Check sheet for the modelled part. Datum: model origin and axes. Units: mm. Face numbers are marked on the shaded views. A direction names the side the tool comes from. Give positions to 0.01 mm unless a question says otherwise; leave off trailing zeros. Order: outer loops, then holes, each group sorted by start corner. A loop starts at its lowest first (then second) coordinate and runs counter-clockwise, first axis right, second up.
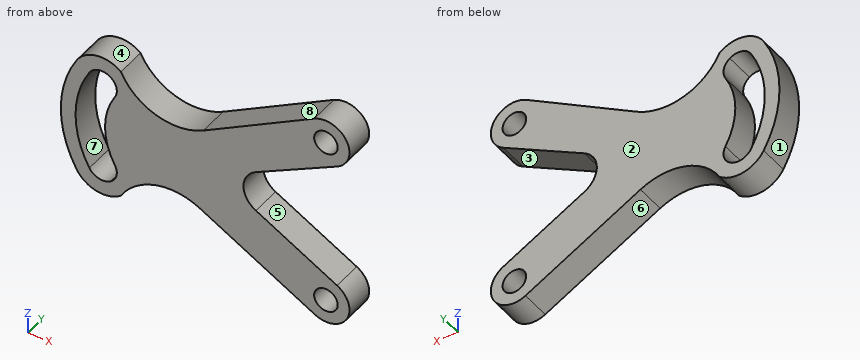
from build123d import *

# Parameters (mm, degrees)
F0_R     = 10
F1_DEPTH = 25


with BuildPart() as f1:
    # F0 (on Front) → F1 (new body)
    with BuildSketch(Plane.XZ):
        with BuildLine():
            Line((65.554609, 17.629084), (134.445391, 54.5397))
            ThreePointArc((134.445391, 54.5397), (142.476996, 81.892703), (115, 89.489292))
            Line((115, 89.489292), (21.000572, 35.218697))
            ThreePointArc((21.000572, 35.218697), (-18.704666, 30.731307), (-49.0183, 56.764481))
            ThreePointArc((-49.0183, 56.764481), (-69.380297, 62.104661), (-86.60254, 50))
            ThreePointArc((-86.60254, 50), (-100, 0), (-86.60254, -50))
            ThreePointArc((-86.60254, -50), (-69.380297, -62.104661), (-49.0183, -56.764481))
            ThreePointArc((-49.0183, -56.764481), (-19.419281, -33.5396), (17.992089, -37.525377))
            Line((17.992089, -37.525377), (115.554609, -89.797867))
            ThreePointArc((115.554609, -89.797867), (142.629084, -81.614174), (134.445391, -54.5397))
            Line((134.445391, -54.5397), (65.554609, -17.629084))
            ThreePointArc((65.554609, -17.629084), (55, 0), (65.554609, 17.629084))
        make_face()
        with BuildLine():
            ThreePointArc((-75.777223, 43.75), (-67.680804, 49.698488), (-57.821535, 47.766831))
            ThreePointArc((-57.821535, 47.766831), (-52.753417, 40.228899), (-54.126588, 31.25))
            ThreePointArc((-54.126588, 31.25), (-62.5, 0), (-54.126588, -31.25))
            ThreePointArc((-54.126588, -31.25), (-52.753417, -40.228899), (-57.821535, -47.766831))
            ThreePointArc((-57.821535, -47.766831), (-67.680804, -49.698488), (-75.777223, -43.75))
            ThreePointArc((-75.777223, -43.75), (-87.5, 0), (-75.777223, 43.75))
        make_face(mode=Mode.SUBTRACT)
        with Locations((125, -72.168784)):
            Circle(F0_R, mode=Mode.SUBTRACT)
        with Locations((125, 72.168784)):
            Circle(F0_R, mode=Mode.SUBTRACT)
    extrude(amount=F1_DEPTH)


solid = f1.part
1) Depth check by flat-ended pin: pin 1 Ø12 at (y, z) = (-21, 52) entering from -X; pin 2 Ø1.5 at (y, z) = (-9.5, 31) entering from -X; pin 3 Ø3 at (x, y) = (-52.5, -10.5) entering from +Z. Enter the tip coordinate at first touch or a pass-through.
Recorded:
pin 1: stops at x = -88.79
pin 2: stops at x = -95.31
pin 3: stops at z = 59.97
2) Section check D-D, the plane x = 27. Record the cut outline in (y, z), then the cut area to 3 significant figures.
Recorded:
outline: (-25, -42.35) - (0, -42.35) - (0, 38.68) - (-25, 38.68) - close
area: 2,030 mm2
3) Section check C-C, the plane x = 70. Record the cut outline in (y, z), then the cut area to 3 significant figures.
Recorded:
outline: (-25, -65.39) - (0, -65.39) - (0, -20.01) - (-25, -20.01) - close; (-25, 20.01) - (0, 20.01) - (0, 63.51) - (-25, 63.51) - close
area: 2,220 mm2
4) Section check B-B, the plane y = -9.75. Record the cut outline in (x, z), then the cut area to 3 significant figures.
Recorded:
outline: (-86.6, -50) arc R25 ccw to (-49.02, -56.76) arc R50 cw to (17.99, -37.53) - (115.55, -89.8) arc R20 ccw to (134.45, -54.54) - (65.55, -17.63) arc R20 cw to (65.55, 17.63) - (134.45, 54.54) arc R20 ccw (long way) to (115, 89.49) - (21, 35.22) arc R50 cw to (-49.02, 56.76) arc R25 ccw to (-86.6, 50) arc R100 ccw to start; hole (-75.78, -43.75) arc R12.5 ccw to (-57.82, -47.77) arc R12.5 ccw to (-54.13, -31.25) arc R62.5 cw to (-54.13, 31.25) arc R12.5 ccw to (-57.82, 47.77) arc R12.5 ccw to (-75.78, 43.75) arc R87.5 ccw to start; hole circle Ø20 at (125, -72.17); hole circle Ø20 at (125, 72.17)
area: 18,100 mm2
5) Set-up check for the marked faces 5, 6, 7 and 8: record each of +Z, -Z, +X, -X, +Y, -Y from which the full face is reachable in a straight line by a thin tool's end or side.
Recorded:
face 5: +X, +Y, -Y
face 6: -Z, +Y, -Y
face 7: +Y, -Y
face 8: +Z, +Y, -Y
6) Section check A-A, the plane x = 125. Record the cut outline in (y, z).
Recorded:
outline: (-25, -92.17) - (0, -92.17) - (0, -82.17) - (-25, -82.17) - close; (-25, -62.17) - (0, -62.17) - (0, -49.48) - (-25, -49.48) - close; (-25, 49.48) - (0, 49.48) - (0, 62.17) - (-25, 62.17) - close; (-25, 82.17) - (0, 82.17) - (0, 92.17) - (-25, 92.17) - close
7) Draft check along Z on the marked faces 1, 2, 3 and 4. Enter one of: +Z half, -Z half, draft (parallel to the pull), parting line (faces both ways), or undercut.
Recorded:
face 1: parting line
face 2: draft
face 3: undercut
face 4: +Z half
8) Material ranges on L1, parallel to Z at x = 125, y = -6.25; L2, parallel to X at y = -14.25, z = -41.5; L3, parallel to X at y = -7.75, z = 35, recorded low to high.
Recorded:
L1: z = -92.17 to -82.17, -62.17 to -49.48, 49.48 to 62.17, 82.17 to 92.17
L2: x = -90.98 to -77.03, -53.11 to -35.49, 25.41 to 110.11
L3: x = -93.67 to -80.2, -52.7 to -28.62, 20.62 to 97.98
